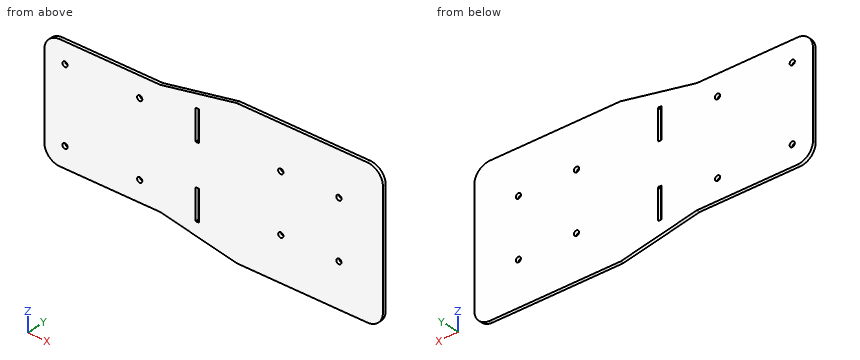
```python
from build123d import *

# Parameters (mm, degrees)
BOSS_EXTRUDE1_DEPTH = 3.175
SKETCH5_R           = 2.5
CUT_EXTRUDE2_DEPTH  = 280.554253455
CUT_EXTRUDE3_DEPTH  = 280.554253455
FILLET1_R           = 15
FILLET2_R           = 5
SKETCH7_R           = 2.5
CUT_EXTRUDE4_DEPTH  = 280.554253455


with BuildPart() as part:
    # Sketch1 → Boss-Extrude1 (new body)
    with BuildSketch(Plane(origin=(0, 0, 0), x_dir=(1, 0, 0), z_dir=(0, 1, 0))):
        Polygon((56, 56), (129.5, 70.5), (270.5, 70.5), (270.5, -70.5), (129.5, -70.5), (56, -56), (-56, -56), (-56, 56), align=None)
    extrude(amount=BOSS_EXTRUDE1_DEPTH)

    # Sketch5 → Cut-Extrude2 (cut, through all)
    with BuildSketch(Plane(origin=(0, 3.175, 0), x_dir=(1, 0, 0), z_dir=(0, 1, 0))):
        with Locations(Location((172, 28, 0), (0, 0, 270))):
            Circle(SKETCH5_R)
        with Locations(Location((228, 28, 0), (0, 0, 90))):
            Circle(SKETCH5_R)
        with Locations(Location((228, -28, 0), (0, 0, 270))):
            Circle(SKETCH5_R)
        with Locations(Location((172, -28, 0), (0, 0, 90))):
            Circle(SKETCH5_R)
    extrude(amount=-CUT_EXTRUDE2_DEPTH, mode=Mode.SUBTRACT)

    # Sketch6 → Cut-Extrude3 (cut, through all)
    with BuildSketch(Plane(origin=(0, 3.175, 0), x_dir=(1, 0, 0), z_dir=(0, 1, 0))):
        with BuildLine():
            Line((93.2, 20.5), (93.2, 49.5))
            ThreePointArc((93.2, 49.5), (93.053553391, 49.853553391), (92.7, 50))
            Line((92.7, 50), (90.5, 50))
            ThreePointArc((90.5, 50), (90.146446609, 49.853553391), (90, 49.5))
            Line((90, 49.5), (90, 20.5))
            ThreePointArc((90, 20.5), (90.146446609, 20.146446609), (90.5, 20))
            Line((90.5, 20), (92.7, 20))
            ThreePointArc((92.7, 20), (93.053553391, 20.146446609), (93.2, 20.5))
        make_face()
        with BuildLine():
            Line((90.5, -20), (92.7, -20))
            ThreePointArc((92.7, -20), (93.053553391, -20.146446609), (93.2, -20.5))
            Line((93.2, -20.5), (93.2, -49.5))
            ThreePointArc((93.2, -49.5), (93.053553391, -49.853553391), (92.7, -50))
            Line((92.7, -50), (90.5, -50))
            ThreePointArc((90.5, -50), (90.146446609, -49.853553391), (90, -49.5))
            Line((90, -49.5), (90, -20.5))
            ThreePointArc((90, -20.5), (90.146446609, -20.146446609), (90.5, -20))
        make_face()
    extrude(amount=-CUT_EXTRUDE3_DEPTH, mode=Mode.SUBTRACT)

    # Fillet1
    fillet1_edges = [part.edges().sort_by_distance(p)[0] for p in [
        (270.5, 1.5875, 70.5),
        (-56, 1.5875, 56),
        (-56, 1.5875, -56),
        (270.5, 1.5875, -70.5),
    ]]
    fillet(fillet1_edges, radius=FILLET1_R)

    # Fillet2
    fillet2_edges = [part.edges().sort_by_distance(p)[0] for p in [
        (129.5, 1.5875, 70.5),
        (56, 1.5875, 56),
        (56, 1.5875, -56),
        (129.5, 1.5875, -70.5),
    ]]
    fillet(fillet2_edges, radius=FILLET2_R)

    # Sketch7 → Cut-Extrude4 (cut, through all)
    with BuildSketch(Plane(origin=(0, 3.175, 0), x_dir=(1, 0, 0), z_dir=(0, 1, 0))):
        with Locations(Location((-36, 36, 0), (0, 0, 270))):
            Circle(SKETCH7_R)
        with Locations(Location((36, 36, 0), (0, 0, 90))):
            Circle(SKETCH7_R)
        with Locations(Location((-36, -36, 0), (0, 0, 90))):
            Circle(SKETCH7_R)
        with Locations(Location((36, -36, 0), (0, 0, 270))):
            Circle(SKETCH7_R)
    extrude(amount=-CUT_EXTRUDE4_DEPTH, mode=Mode.SUBTRACT)


solid = part.part
```
The model under review builds one solid part; all positions refer to its coordinate system, in mm. Round coordinates to 2 decimals unless told otherwise and drop trailing zeros. Loops run counter-clockwise (first coordinate to the right, second up) from the corner with the lowest first, then second, coordinate; pieces in that order, holes last. Notation, with made-up numbers: M 37.25,9.5 L 70.25,9.5 A18 cw 70.25,36.5 Z; hole C 60.5,-1 d5. An arc over 180 degrees is marked long. Write item = value, one per line.
Item 1: Take a section at A-A on y = 2.5. State how many separate pieces and enclosed holes the cut face has, then the cut area to 3 significant figures.
Return value:
separate_pieces = 1
enclosed_holes = 10
area = 41,200 mm2
Item 2: Insertion check: P1, Ø3, axis at x = -36, z = -36, coming from the +Y side; P2, Ø1, axis at x = 5.5, y = 2, coming from the -Z side; P3, Ø1.1, axis at x = 91, y = 1.5, coming from the +Z side; P4, Ø1.1, axis at x = 91.5, y = 2, coming from the +Z side. Each pin has a flat end and moves straight along its axis. Give the tip position at first contact, or say it passes through.
Return value:
P1 = through
P2 = -56
P3 = 63.01
P4 = 63.11
Item 3: For line 1 (X direction, y = 1.9, z = 36); line 2 (X direction, y = 0.9, z = -28); line 3 (Z direction, x = 228, y = 0.7), list the stretches that pass through material, from the lowest coordinate up. Write a range as [from, to].
Return value:
line_1 = [-56, -38.5], [-33.5, 33.5], [38.5, 90], [93.2, 270.5]
line_2 = [-56, 90], [93.2, 169.5], [174.5, 225.5], [230.5, 270.5]
line_3 = [-70.5, -30.5], [-25.5, 25.5], [30.5, 70.5]
Item 4: Take a section at B-B on x = 11. Write out the cut boundary in (y, z) (3 decimals).
Return value:
outline = M 0,-56 L 3.175,-56 L 3.175,56 L 0,56 Z
Item 5: Take a section at C-C on x = 111. Write out the cut boundary in (y, z) (3 decimals), then the cut area to 4 significant figures.
Return value:
outline = M 0,-66.85 L 3.175,-66.85 L 3.175,66.85 L 0,66.85 Z
area = 424.5 mm2
